from build123d import *

# Parameters (mm, degrees)
SKETCH_1_W          = 35
SKETCH_1_H          = 90
EXTRUDE_1_DEPTH     = 5
SKETCH_2_W          = 35
SKETCH_2_H          = 17
EXTRUDE_2_DEPTH     = 9
FILLET_1_R          = 7
SKETCH_3_R          = 1.5
CUT_EXTRUDE_3_DEPTH = 51.271761457
CUT_EXTRUDE_4_DEPTH = 51.271761457
FILLET_2_R          = 2


with BuildPart() as part:
    # 草图1 → 凸台-拉伸1 (new body)
    with BuildSketch(Plane.XY):
        Rectangle(SKETCH_1_W, SKETCH_1_H)
    extrude(amount=EXTRUDE_1_DEPTH)

    # 草图2 → 凸台-拉伸2 (add)
    with BuildSketch(Plane.XY.offset(5)):
        with Locations((0, -36.5)):
            Rectangle(SKETCH_2_W, SKETCH_2_H)
    extrude(amount=EXTRUDE_2_DEPTH)

    # 圆角1
    fillet_1_edges = [part.edges().sort_by_distance(p)[0] for p in [
        (0, -28, 5),
    ]]
    fillet(fillet_1_edges, radius=FILLET_1_R)

    # 草图3 → 切除-拉伸3 (cut, through all)
    with BuildSketch(Plane.XY.offset(14)):
        with Locations((-7.5, -37.5)):
            Circle(SKETCH_3_R)
        with Locations((7.5, -37.5)):
            Circle(SKETCH_3_R)
    extrude(amount=-CUT_EXTRUDE_3_DEPTH, mode=Mode.SUBTRACT)

    # 草图4 → 切除-拉伸4 (cut, through all)
    with BuildSketch(Plane(origin=(0, 0, 0), x_dir=(-1, 0, 0), z_dir=(0, 0, -1))):
        Polygon((-17.5, 29), (-17.5, 21), (-7.5, 21), align=None)
    extrude(amount=-CUT_EXTRUDE_4_DEPTH, mode=Mode.SUBTRACT)

    # 圆角2
    fillet_2_edges = [part.edges().sort_by_distance(p)[0] for p in [
        (7.5, 21, 2.5),
    ]]
    fillet(fillet_2_edges, radius=FILLET_2_R)


solid = part.part
Verification items for the finished model (mm, model axes). A direction names the side the tool comes from. Coordinates: 2 decimals unless noted, no trailing zeros. Order: outer loops, then holes, each group sorted by start corner. A loop starts at its lowest first (then second) coordinate and runs counter-clockwise, first axis right, second up.
1. Sectioned sample at D-D, the plane z = 9.5. Record the cut outline in (x, y).
Results found:
outline: (-17.5, -45) - (17.5, -45) - (17.5, -27.54) - (-17.5, -27.54) - close; hole circle Ø3 at (-7.5, -37.5); hole circle Ø3 at (7.5, -37.5)
2. Sectioned sample at B-B, the plane x = -7.5. Record the cut outline in (y, z).
Results found:
outline: (-45, 0) - (-39, 0) - (-39, 14) - (-45, 14) - close; (-36, 0) - (45, 0) - (45, 5) - (-21, 5) arc R7 cw to (-28, 12) - (-28, 14) - (-36, 14) - close
3. Go/stop test with flat-tipped pins: pin 1 Ø4 at (x, y) = (8.5, 30.5) entering from -Z; pin 2 Ø4 at (x, y) = (8, -7.5) entering from +Z; pin 3 Ø0.6 at (x, z) = (-2.5, 13) entering from +Y; pin 4 Ø1.5 at (x, z) = (-11, 7.5) entering from +Y. Record where each tip stops, or that it passes through.
Results found:
pin 1: stops at z = 0
pin 2: stops at z = 5
pin 3: stops at y = -28
pin 4: stops at y = -25.63
4. Release check for a two-part mould opening along Y. For faces 1 (the face through (17.5, 37, 2)), 2 (the face through (11.303, 22.371, 2.535)), 3 (the face through (7.175, -38.964, 7.098)), 4 (the face through (0, 45, 2)) record: +Y half, -Y half, draft (parallel to the pull), parting line (faces both ways), or undercut.
Results found:
face 1: draft
face 2: undercut
face 3: undercut
face 4: +Y half
5. Scan lines: line 1 (Z direction, x = -8.5, y = 19.5); line 2 (Y direction, x = -7.5, z = 10); line 3 (Y direction, x = -7.5, z = 10.75). Record each from-to range of solid material in increasing order.
Results found:
line 1: z = 0 to 5
line 2: y = -45 to -39, -36 to -27.71
line 3: y = -45 to -39, -36 to -27.89
6. Sectioned sample at A-A, the plane y = -37.5. Record the cut outline in (x, z).
Results found:
outline: (-17.5, 0) - (-9, 0) - (-9, 14) - (-17.5, 14) - close; (-6, 0) - (6, 0) - (6, 14) - (-6, 14) - close; (9, 0) - (17.5, 0) - (17.5, 14) - (9, 14) - close
7. Set-up check for faces 5 (the face through (0, 12, 5)), 6 (the face through (17.5, -20, 4)), 7 (the face through (15, 27, 2)): record each of +Z, -Z, +X, -X, +Y, -Y from which the full face is reachable in a straight line by a thin tool's end or side.
Results found:
face 5: +Z, +X, -X, +Y
face 6: +Z, -Z, +X, +Y, -Y
face 7: +Z, -Z, +X
8. Sectioned sample at C-C, the plane x = -13. Record the cut outline in (y, z), and give its area (3 significant figures).
Results found:
outline: (-45, 0) - (45, 0) - (45, 5) - (-21, 5) arc R7 cw to (-28, 12) - (-28, 14) - (-45, 14) - close
area: 614 mm2
